```python
from build123d import *

# Parameters (mm, degrees)
SKETCH1_R           = 23.7871
BOSS_EXTRUDE1_DEPTH = 7.0612
SKETCH3_R           = 1.7653
SKETCH5_R           = 1.575
CUT_EXTRUDE1_DEPTH  = 7.0612
BOSS_EXTRUDE3_DEPTH = 7.0612
CUT_EXTRUDE2_DEPTH  = 10
CHAMFER1_SIZE       = 3.5
CHAMFER2_SIZE       = 3.5
CHAMFER3_SIZE       = 3.5
CHAMFER4_SIZE       = 3.5
CHAMFER5_SIZE       = 3.5
CHAMFER6_SIZE       = 3.5


with BuildPart() as part:
    # Sketch1 → Boss-Extrude1 (new body)
    with BuildSketch(Plane(origin=(0, 0, 0), x_dir=(1, 0, 0), z_dir=(0, 1, 0))):
        with Locations(Location((0, 0, 0), (0, 0, 270))):
            Circle(SKETCH1_R)
    extrude(amount=BOSS_EXTRUDE1_DEPTH)

    # Sketch3 → Cut-Revolve1 (revolve, cut)
    with BuildSketch(Plane(origin=(0, 0, 0), x_dir=(0, 0, -1), z_dir=(1, 0, 0))):
        with Locations((23.7871, 3.5306)):
            Circle(SKETCH3_R)
    revolve(axis=Axis((0, 3.5306, 0), (0, 1, 0)), mode=Mode.SUBTRACT)

    # Sketch5 → Cut-Extrude1 (cut)
    with BuildSketch(Plane.XZ):
        with Locations(Location((0, 0, 0), (0, 0, 270))):
            Circle(SKETCH5_R)
    extrude(amount=-CUT_EXTRUDE1_DEPTH, mode=Mode.SUBTRACT)

    # Sketch8 → Boss-Extrude3 (add)
    with BuildSketch(Plane.XZ):
        with BuildLine():
            ThreePointArc((-1.173935688, -1.05), (0, -1.575), (1.173935688, -1.05))
            Line((1.173935688, -1.05), (-1.173935688, -1.05))
        make_face()
    extrude(amount=-BOSS_EXTRUDE3_DEPTH)

    # Sketch18 → Cut-Extrude2 (cut)
    with BuildSketch(Plane(origin=(0, 7.0612, 0), x_dir=(1, 0, 0), z_dir=(0, 1, 0))):
        with BuildLine():
            Line((-8.82820323, 0.709103466), (-13.591342951, 3.459103466))
            ThreePointArc((-13.591342951, 3.459103466), (-17.51207526, 3.056828066), (-20, 0))
            ThreePointArc((-20, 0), (-17.320508076, -10), (-10, -17.320508076))
            ThreePointArc((-10, -17.320508076), (-6.10874687, -16.694316081), (-3.8, -13.5))
            Line((-3.8, -13.5), (-3.8, -8))
            ThreePointArc((-3.8, -8), (-5.147302995, -2.97179677), (-8.82820323, 0.709103466))
        make_face()
        with BuildLine():
            Line((3.8, -8), (3.8, -13.5))
            ThreePointArc((3.8, -13.5), (6.10874687, -16.694316081), (10, -17.320508076))
            ThreePointArc((10, -17.320508076), (17.320508076, -10), (20, 0))
            ThreePointArc((20, 0), (17.51207526, 3.056828066), (13.591342951, 3.459103466))
            Line((13.591342951, 3.459103466), (8.82820323, 0.709103466))
            ThreePointArc((8.82820323, 0.709103466), (5.147302995, -2.97179677), (3.8, -8))
        make_face()
        with BuildLine():
            Line((5.02820323, 7.290896534), (9.791342951, 10.040896534))
            ThreePointArc((9.791342951, 10.040896534), (11.40332839, 13.637488015), (10, 17.320508076))
            ThreePointArc((10, 17.320508076), (0, 20), (-10, 17.320508076))
            ThreePointArc((-10, 17.320508076), (-11.40332839, 13.637488015), (-9.791342951, 10.040896534))
            Line((-9.791342951, 10.040896534), (-5.02820323, 7.290896534))
            ThreePointArc((-5.02820323, 7.290896534), (0, 5.943593539), (5.02820323, 7.290896534))
        make_face()
    extrude(amount=-CUT_EXTRUDE2_DEPTH, mode=Mode.SUBTRACT)

    # Chamfer1
    chamfer1_edges = [part.edges().sort_by_distance(p)[0] for p in [
        (-17.51207526, 7.0612, -3.056828066),
    ]]
    chamfer(chamfer1_edges, length=CHAMFER1_SIZE)
    chamfer1_2_edges = [part.edges().sort_by_distance(p)[0] for p in [
        (-6.10874687, 7.0612, 16.694316081),
    ]]
    chamfer(chamfer1_2_edges, length=CHAMFER1_SIZE)
    chamfer1_3_edges = [part.edges().sort_by_distance(p)[0] for p in [
        (-11.209773091, 7.0612, -2.084103466),
        (-3.8, 7.0612, 10.75),
        (-5.147302995, 7.0612, 2.97179677),
    ]]
    chamfer(chamfer1_3_edges, length=CHAMFER1_SIZE)
    chamfer1_4_edges = [part.edges().sort_by_distance(p)[0] for p in [
        (-17.320508076, 7.0612, 10),
    ]]
    chamfer(chamfer1_4_edges, length=CHAMFER1_SIZE - 0.0001)  # a hair under: the kernel refuses the full size

    # Chamfer2
    chamfer2_edges = [part.edges().sort_by_distance(p)[0] for p in [
        (-11.40332839, 7.0612, -13.637488015),
    ]]
    chamfer(chamfer2_edges, length=CHAMFER2_SIZE)
    chamfer2_2_edges = [part.edges().sort_by_distance(p)[0] for p in [
        (11.40332839, 7.0612, -13.637488015),
    ]]
    chamfer(chamfer2_2_edges, length=CHAMFER2_SIZE)
    chamfer2_3_edges = [part.edges().sort_by_distance(p)[0] for p in [
        (7.409773091, 7.0612, -8.665896534),
        (0, 7.0612, -5.943593539),
        (-7.409773091, 7.0612, -8.665896534),
    ]]
    chamfer(chamfer2_3_edges, length=CHAMFER2_SIZE)
    chamfer2_4_edges = [part.edges().sort_by_distance(p)[0] for p in [
        (0, 7.0612, -20),
    ]]
    chamfer(chamfer2_4_edges, length=CHAMFER2_SIZE - 0.0001)  # a hair under: the kernel refuses the full size

    # Chamfer3
    chamfer3_edges = [part.edges().sort_by_distance(p)[0] for p in [
        (17.51207526, 7.0612, -3.056828066),
    ]]
    chamfer(chamfer3_edges, length=CHAMFER3_SIZE)
    chamfer3_2_edges = [part.edges().sort_by_distance(p)[0] for p in [
        (6.10874687, 7.0612, 16.694316081),
    ]]
    chamfer(chamfer3_2_edges, length=CHAMFER3_SIZE)
    chamfer3_3_edges = [part.edges().sort_by_distance(p)[0] for p in [
        (5.147302995, 7.0612, 2.97179677),
        (11.209773091, 7.0612, -2.084103466),
        (3.8, 7.0612, 10.75),
    ]]
    chamfer(chamfer3_3_edges, length=CHAMFER3_SIZE - 0.0001)  # a hair under: the kernel refuses the full size
    chamfer3_4_edges = [part.edges().sort_by_distance(p)[0] for p in [
        (17.320508076, 7.0612, 10),
    ]]
    chamfer(chamfer3_4_edges, length=CHAMFER3_SIZE - 0.0001)  # a hair under: the kernel refuses the full size

    # Chamfer4
    chamfer4_edges = [part.edges().sort_by_distance(p)[0] for p in [
        (17.51207526, 0, -3.056828066),
    ]]
    chamfer(chamfer4_edges, length=CHAMFER4_SIZE)
    chamfer4_2_edges = [part.edges().sort_by_distance(p)[0] for p in [
        (6.10874687, 0, 16.694316081),
    ]]
    chamfer(chamfer4_2_edges, length=CHAMFER4_SIZE)
    chamfer4_3_edges = [part.edges().sort_by_distance(p)[0] for p in [
        (17.320508076, 0, 10),
    ]]
    chamfer(chamfer4_3_edges, length=CHAMFER4_SIZE - 0.0001)  # a hair under: the kernel refuses the full size
    chamfer4_4_edges = [part.edges().sort_by_distance(p)[0] for p in [
        (11.209773091, 0, -2.084103466),
        (3.8, 0, 10.75),
        (5.147302995, 0, 2.97179677),
    ]]
    chamfer(chamfer4_4_edges, length=CHAMFER4_SIZE)

    # Chamfer5
    chamfer5_edges = [part.edges().sort_by_distance(p)[0] for p in [
        (-11.40332839, 0, -13.637488015),
    ]]
    chamfer(chamfer5_edges, length=CHAMFER5_SIZE)
    chamfer5_2_edges = [part.edges().sort_by_distance(p)[0] for p in [
        (11.40332839, 0, -13.637488015),
    ]]
    chamfer(chamfer5_2_edges, length=CHAMFER5_SIZE)
    chamfer5_3_edges = [part.edges().sort_by_distance(p)[0] for p in [
        (7.409773091, 0, -8.665896534),
        (0, 0, -5.943593539),
        (-7.409773091, 0, -8.665896534),
    ]]
    chamfer(chamfer5_3_edges, length=CHAMFER5_SIZE)
    chamfer5_4_edges = [part.edges().sort_by_distance(p)[0] for p in [
        (0, 0, -20),
    ]]
    chamfer(chamfer5_4_edges, length=CHAMFER5_SIZE - 0.0001)  # a hair under: the kernel refuses the full size

    # Chamfer6
    chamfer6_edges = [part.edges().sort_by_distance(p)[0] for p in [
        (-6.10874687, 0, 16.694316081),
    ]]
    chamfer(chamfer6_edges, length=CHAMFER6_SIZE)
    chamfer6_2_edges = [part.edges().sort_by_distance(p)[0] for p in [
        (-17.51207526, 0, -3.056828066),
    ]]
    chamfer(chamfer6_2_edges, length=CHAMFER6_SIZE)
    chamfer6_3_edges = [part.edges().sort_by_distance(p)[0] for p in [
        (-11.209773091, 0, -2.084103466),
        (-5.147302995, 0, 2.97179677),
        (-3.8, 0, 10.75),
    ]]
    chamfer(chamfer6_3_edges, length=CHAMFER6_SIZE)
    chamfer6_4_edges = [part.edges().sort_by_distance(p)[0] for p in [
        (-17.320508076, 0, 10),
    ]]
    chamfer(chamfer6_4_edges, length=CHAMFER6_SIZE - 0.0001)  # a hair under: the kernel refuses the full size


solid = part.part
```
Work out the finished part from the listing and answer in its coordinate system (mm). A direction names the side the tool comes from. Give positions to 0.01 mm unless a question says otherwise; leave off trailing zeros. Loops run counter-clockwise (first coordinate to the right, second up) from the corner with the lowest first, then second, coordinate; pieces in that order, holes last. Notation, with made-up numbers: (-15.75, 5) -> (-9.75, 5) arc R12 cw to (-9.75, 20) -> close; hole circle Ø6 at (68.5, 70.5). An arc over 180 degrees is marked (long way). Write item = value, one per line. Start each with the question number.
(1) Find the intervals of material crossed by probe 1 along Z at (x, y) = (6, 6.5); probe 2 along X at (y, z) = (6, 16.5); probe 3 along X at (y, z) = (5.5, 0) (3 decimals), in increasing order. Write a range as from..to.
(2) Which of the six approach directions +Z, -Z, +X, -X, +Y, -Y give full straight-line access (tool end or side, diameter ignored) to faces 3 (the conical face through (-3.948, 2.163, 2.376)), 4 (the conical face through (12.74, 4.9, -13.56)), 5 (the flat face through (0, 3, -1.05))?
(3) Find section A-A on y = 2.5. Give the vertices of the cut face in (x, z) (3 decimals), and give its area (3 significant figures).
(4) Find section B-B on z = 11.5. Give the number of separate pieces and of enclosed holes in the cut face, and give its area (3 significant figures).
(5) Given pin 1 Ø1.5 at (x, y) = (10, 6) entering from +Z; pin 2 Ø2 at (x, y) = (8.5, 4.5) entering from -Z; pin 3 Ø1.9 at (x, y) = (-0.5, 3.5) entering from +Z, each flat-ended and moving along its own axis, determine where each tip first touches the part or whether it passes through.
(6) The mould has two halves that part along X. Classify faces 1 (the flat face through (-2.1, 1.8, 11)), 2 (the cylindrical face through (-23.22, 6.17, -5.16)): +X half, -X half, draft (parallel to the pull), parting line (faces both ways), or undercut.
From the geometry:
q1.probe_1 = -23.02..-22.14, -4.47..-2.35, 19.89..23.02
q1.probe_2 = -17.13..-15.21, -2.48..2.48, 15.21..17.13
q1.probe_3 = -23.787..-21.939, -4.919..-1.575, 1.575..4.919, 21.939..23.787
q2.face_3 = -Y
q2.face_4 = +Y
q2.face_5 = +Y, -Y
q3.outline = circle Ø44.708 at (0, 0); hole (-20.999, -0.142) arc R6.15 ccw to (-13.188, -4.381) -> (-8.328, -1.575) arc R11.056 ccw to (-2.8, 8) -> (-2.8, 13.612) arc R6.15 ccw to (-10.377, 18.257) arc R21 ccw to start; hole (-10.622, -18.115) arc R21 ccw to (10.622, -18.115) arc R6.15 ccw to (10.388, -9.231) -> (5.528, -6.425) arc R11.056 ccw to (-5.528, -6.425) -> (-10.388, -9.231) arc R6.15 ccw to start; hole (-1.174, -1.05) -> (1.174, -1.05) arc R1.575 ccw (long way) to start; hole (2.8, 8) arc R11.056 ccw to (8.328, -1.575) -> (13.188, -4.381) arc R6.15 ccw to (20.999, -0.142) arc R21 ccw to (10.377, 18.257) arc R6.15 ccw to (2.8, 13.612) -> close
q3.area = 641 mm^2
q4.separate_pieces = 3
q4.enclosed_holes = 0
q4.area = 51.6 mm^2
q5.pin_1 = 21.91
q5.pin_2 = -22.44
q5.pin_3 = 22.31
q6.face_1 = undercut
q6.face_2 = parting line
